from build123d import *

# Parameters (mm, degrees)
SKETCH1_R                = 21.4
SKETCH1_R_2              = 20.5
SKETCH1_R_3              = 1.55
BOSS_EXTRUDE1_DEPTH      = 11.5
SKETCH1_3_R              = 1.55
BOSS_EXTRUDE2_DEPTH      = 11.5
BOSS_EXTRUDE2_DEPTH_BACK = 5


with BuildPart() as part:
    # Sketch1 → Boss-Extrude1 (new body)
    with BuildSketch(Plane(origin=(0, 0, 0), x_dir=(1, 0, 0), z_dir=(0, 1, 0))):
        with Locations(Location((0, 0, 0), (0, 0, 270))):
            Circle(SKETCH1_R)
        Circle(SKETCH1_R_2, mode=Mode.SUBTRACT)
        Circle(SKETCH1_R_2)
        with Locations(Location((-8.6, 0, 0), (0, 0, 270))):
            Circle(SKETCH1_R_3, mode=Mode.SUBTRACT)
        with Locations(Location((8.6, 0, 0), (0, 0, 270))):
            Circle(SKETCH1_R_3, mode=Mode.SUBTRACT)
    extrude(amount=BOSS_EXTRUDE1_DEPTH)

    # Sketch1_3 → Boss-Extrude2 (add, two sides)
    with BuildSketch(Plane(origin=(0, 0, 0), x_dir=(1, 0, 0), z_dir=(0, 1, 0))) as boss_extrude2_sk:
        with Locations(Location((-8.6, 0, 0), (0, 0, 270))):
            Circle(SKETCH1_3_R)
        with Locations(Location((8.6, 0, 0), (0, 0, 270))):
            Circle(SKETCH1_3_R)
    extrude(amount=BOSS_EXTRUDE2_DEPTH)
    extrude(boss_extrude2_sk.sketch, amount=-BOSS_EXTRUDE2_DEPTH_BACK)


solid = part.part
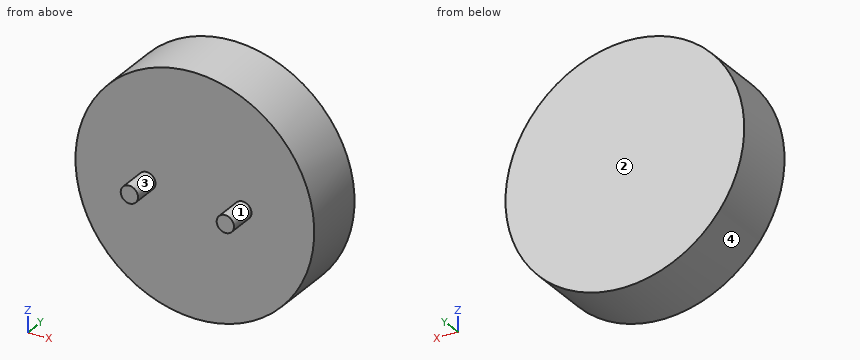
For this review, take the finished solid that the model builds, in its own axes (mm). Face numbers are marked on the shaded views. Round coordinates to 2 decimals unless told otherwise and drop trailing zeros. Write each loop counter-clockwise with the first axis right and the second up, starting at its lowest first coordinate (ties: lowest second). Pieces come first, ordered by that corner, then holes. Notation, with made-up numbers: M 70.25,13 L 110.25,13 A20 ccw 110.25,43 Z; hole C -8.5,-40 d3. An arc over 180 degrees is marked long. Write item = value, one per line. Start each with the question number.
(1) We need section A-A (y = -1.25). Give the boundary of the cut face in (x, z).
(2) For line 1 along Y through (x, z) = (14, 1.5); line 2 along X through (y, z) = (-1, 0.5); line 3 along Z through (x, y) = (11.5, 5.5), list the stretches that pass through material, from the lowest coordinate up.
(3) We need section B-B (z = 0). Give the boundary of the cut face in (x, y).
(4) Clearance check with flat-ended pins moving along their axes: pin 1 Ø1.5 at (x, y) = (-1, 7) entering from -Z; pin 2 Ø5 at (x, z) = (-3, -7) entering from -Y; pin 3 Ø4 at (y, z) = (3.5, 10.5) entering from +X. State where each tip first meets the part, or that it passes through.
(5) We need section C-C (x = 0). Give the boundary of the cut face in (y, z), then the cut area to 3 significant figures.
(6) We need section D-D (y = 2.25). Give the boundary of the cut face in (x, z).
(7) The part is to be moulded in two halves that separate along X. For the marked faces 1, 2, 3 and 4, say which applies: +X half, -X half, draft (parallel to the pull), parting line (faces both ways), or undercut.
Results found:
q1.outline = C -8.6,0 d3.1; C 8.6,0 d3.1
q2.line_1 = 0 to 11.5
q2.line_2 = -10.07 to -7.13, 7.13 to 10.07
q2.line_3 = -18.05 to 18.05
q3.outline = M -21.4,0 L -10.15,0 L -10.15,-5 L -7.05,-5 L -7.05,0 L 7.05,0 L 7.05,-5 L 10.15,-5 L 10.15,0 L 21.4,0 L 21.4,11.5 L -21.4,11.5 Z
q4.pin_1 = -21.4
q4.pin_2 = 0
q4.pin_3 = 19.64
q5.outline = M 0,-21.4 L 11.5,-21.4 L 11.5,21.4 L 0,21.4 Z
q5.area = 492 mm²
q6.outline = C 0,0 d42.8
q7.face_1 = undercut
q7.face_2 = draft
q7.face_3 = undercut
q7.face_4 = parting line
